Autodesk Inventor part; units mm, degrees
ref_plane "YZ Plane" through (0, 0, 0) normal (1, 0, 0) x (0, 1, 0)
ref_plane "XZ Plane" through (0, 0, 0) normal (0, 1, 0) x (-1, 0, 0)
ref_plane "XY Plane" through (0, 0, 0) normal (0, 0, 1) x (1, 0, 0)
sketch "スケッチ1" plane through (0, 0, 0) normal (0, 0, 1) x (1, 0, 0)
  line L0 (-100, -100) -> (100, -100)
  line L1 (100, -100) -> (100, 100)
  line L2 (100, 100) -> (-100, 100)
  line L3 (-100, 100) -> (-100, -100)
  line L4 (-100, -100) -> (100, 100) construction
  line L5 (100, -100) -> (-100, 100) construction
  point P0 (0, 0)
  dimension "d0" = 200
  dimension "d1" = 200
extrude "押し出し1" add sketch "スケッチ1" along normal blind 2
sketch "スケッチ2" plane through (0, 0, 2) normal (0, 0, 1) x (1, 0, 0)
  line L0 (100, 100) -> (-100, 100)
  line L1 (100, 100) -> (70, 100)
  line L2 (70, 100) -> (70, 70)
  line L3 (70, 70) -> (100, 70)
  line L4 (100, 70) -> (100, 100)
  line L5 (-100, -100) -> (100, -100)
  line L6 (-100, 100) -> (-100, -100)
  line L7 (-100, 100) -> (-70, 100)
  line L8 (-70, 100) -> (-70, 70)
  line L9 (-70, 70) -> (-100, 70)
  line L10 (-100, 70) -> (-100, 100)
  point P0 (0, 0)
  point P1 (-100, 70)
  dimension "d4" = 170
  dimension "d5" = 30
  dimension "d6" = 30
  dimension "d7" = 170
extrude "押し出し2" cut sketch "スケッチ2" against normal blind 2
sketch "スケッチ3" plane through (0, 0, 0) normal (0, 0, -1) x (-1, 0, 0)
  line L0 (-70, 100) -> (70, 100)
  point P0 (0, 0)
  point P1 (-35.7932, 78)
  point P2 (37.7411, 78)
  point P3 (-61, 89.1596)
  point P4 (61, 89.1596)
  point P5 (-50, 82.5)
  point P6 (-30, 82.5)
  point P7 (-10, 82.5)
  point P8 (0.0001, 82.5183)
  point P9 (10, 82.5545)
  point P10 (30, 82.5545)
  point P11 (50, 82.5545)
  point P12 (51.6496, 93.6869)
  dimension "d10" = 22
  dimension "d11" = 61
  dimension "d12" = 61
  dimension "d13" = 17.5
  dimension "d14" = 11
  dimension "d15" = 31
  dimension "d16" = 51
  dimension "d17" = 71
  dimension "d18" = 91
  dimension "d19" = 111
hole "穴1" at (50, 82.5, 0) at (30, 82.5, 0) at (10, 82.5, 0) at (-10, 82.5545, 0) at (-30, 82.5545, 0) at (-50, 82.5545, 0) at (-0.0001, 82.5183, 0) direction (0, 0, 1) diameter 3.4 end through all
sketch "スケッチ4" plane through (0, 0, 0) normal (0, 0, -1) x (-1, 0, 0)
  line L0 (-70, 70) -> (-100, 70)
  line L1 (-100, -100) -> (-100, 70)
  line L2 (100, 70) -> (100, -100)
  line L3 (100, 70) -> (70, 70)
  point P0 (0, 0)
  point P1 (-90, 55)
  point P2 (-66, 55)
  point P3 (-90, 25)
  point P4 (-66, 25)
  point P5 (90, 58)
  point P6 (66, 58)
  point P7 (90, 12.16)
  point P8 (66, 12.16)
  dimension "d27" = 15
  dimension "d28" = 15
  dimension "d29" = 10
  dimension "d30" = 24
  dimension "d31" = 10
  dimension "d32" = 30
  dimension "d33" = 30
  dimension "d34" = 24
  dimension "d35" = 10
  dimension "d36" = 12
  dimension "d37" = 24
  dimension "d38" = 10
  dimension "d39" = 24
hole "穴2" at (66, 25, 0) at (90, 25, 0) at (66, 55, 0) at (90, 55, 0) direction (0, 0, 1) diameter 3.4 end through all
sketch "スケッチ5" plane through (0, 0, 0) normal (0, 0, -1) x (-1, 0, 0)
  point P0 (0, 0)
sketch "スケッチ6" plane through (0, 0, 0) normal (0, 0, -1) x (-1, 0, 0)
  line L0 (100, 70) -> (70, 70)
  line L1 (100, 70) -> (100, -100)
  point P0 (0, 0)
  point P1 (90, 55)
  point P2 (66, 55)
  point P3 (90, 25)
  point P4 (66, 25)
  dimension "d47" = 15
  dimension "d48" = 15
  dimension "d49" = 10
  dimension "d50" = 24
  dimension "d51" = 10
  dimension "d52" = 24
  dimension "d53" = 30
  dimension "d54" = 30
hole "穴3" at (-90, 25, 0) at (-66, 25, 0) at (-66, 55, 0) at (-90, 55, 0) direction (0, 0, 1) diameter 3.4 end through all
sketch "スケッチ7" plane through (0, 0, 0) normal (0, 0, -1) x (-1, 0, 0)
  point P0 (0, 0)
sketch "スケッチ8" plane through (0, 0, 0) normal (0, 0, -1) x (-1, 0, 0)
  line L0 (-100, -100) -> (-100, 70)
  line L1 (-70, 70) -> (-100, 70)
  line L2 (100, 70) -> (70, 70)
  line L3 (100, 70) -> (100, -100)
  point P0 (0, 0)
  point P1 (-95, 65)
  point P2 (95, 65)
  dimension "d62" = 5
  dimension "d63" = 5
  dimension "d64" = 5
  dimension "d65" = 5
hole "穴4" at (95, 65, 0) at (-95, 65, 0) direction (0, 0, 1) diameter 3.4 end through all
sketch "スケッチ9" plane through (0, 0, 0) normal (0, 0, -1) x (-1, 0, 0)
  line L0 (-100, -100) -> (-100, 70)
  line L1 (100, -100) -> (-100, -100)
  line L2 (100, 70) -> (100, -100)
  point P0 (0, 0)
  point P1 (-95, -95)
  point P2 (95, -95)
  dimension "d73" = 5
  dimension "d74" = 5
  dimension "d75" = 5
  dimension "d76" = 5
hole "穴5" at (95, -95, 0) at (-95, -95, 0) direction (0, 0, 1) diameter 3.4 end through all
sketch "スケッチ10" plane through (0, 0, 0) normal (0, 0, -1) x (-1, 0, 0)
  circle A0 centre (-95, 65) radius 1.7
  line L0 (-100, -100) -> (-100, 70)
  line L1 (100, 70) -> (100, -100)
  point P0 (0, 0)
  point P1 (-95, -15)
  point P2 (95, -25)
  dimension "d84" = 80
  dimension "d85" = 5
  dimension "d86" = 5
hole "穴6" at (95, -15, 0) direction (0, 0, 1) diameter 3.4 end through all
sketch "スケッチ11" plane through (0, 0, 0) normal (0, 0, -1) x (-1, 0, 0)
  line L0 (-70, 100) -> (70, 100)
  point P0 (0, 0)
  point P1 (0, 0)
  point P2 (0, -10)
  dimension "d94" = 110
hole "穴7" at (0, -10, 0) direction (0, 0, 1) diameter 3.4 end through all
sketch "スケッチ12" plane through (0, 0, 0) normal (0, 0, -1) x (-1, 0, 0)
  line L0 (100, -100) -> (-100, -100)
  line L1 (100, 70) -> (100, -100)
  line L2 (-100, -100) -> (-100, 70)
  point P0 (0, 0)
  point P1 (-95, -80)
  point P2 (95, -80)
  dimension "d102" = 20
  dimension "d103" = 20
  dimension "d104" = 5
  dimension "d105" = 5
hole "穴8" at (95, -80, 0) at (-95, -80, 0) direction (0, 0, 1) diameter 3.4 end through all
sketch "スケッチ13" plane through (0, 0, 0) normal (0, 0, -1) x (-1, 0, 0)
  point P0 (0, 0)
sketch "スケッチ14" plane through (0, 0, 0) normal (0, 0, -1) x (-1, 0, 0)
  line L0 (100, 70) -> (100, -100)
  circle A0 centre (95, 65) radius 1.7
  point P0 (0, 0)
  point P1 (95, -15)
  dimension "d113" = 5
  dimension "d114" = 80
hole "穴9" at (-95, -15, 0) direction (0, 0, 1) diameter 3.4 end through all
sketch "スケッチ15" plane through (0, 0, 0) normal (0, 0, -1) x (-1, 0, 0)
  circle A0 centre (0, -10) radius 1.7
  point P0 (0, 0)
  point P1 (0, -3)
  dimension "d122" = 7
hole "穴10" at (0, -3, 0) direction (0, 0, 1) diameter 3.4 end through all
sketch "スケッチ16" plane through (0, 0, 2) normal (0, 0, 1) x (1, 0, 0)
  point P0 (0, 0)
  point P1 (-5, 24.9689)
  point P2 (5, 25)
  point P3 (5, 35)
  point P4 (-5, 34.9689)
  dimension "d130" = 5
  dimension "d131" = 5
  dimension "d132" = 10
  dimension "d133" = 10
  dimension "d134" = 5
  dimension "d135" = 5
hole "穴11" at (-5, 34.9689, 2) at (-5, 24.9689, 2) at (5, 25, 2) at (5, 35, 2) direction (0, 0, -1) diameter 2.459 depth 8.8 tip angle 118
sketch "スケッチ17" plane through (0, 0, 2) normal (0, 0, 1) x (1, 0, 0)
  point P0 (0, 0)
properties part number "20220522"
Part model, mm, in its own coordinate system. Give positions to 0.01 mm unless a question says otherwise; leave off trailing zeros. Loops run counter-clockwise (first coordinate to the right, second up) from the corner with the lowest first, then second, coordinate; pieces in that order, holes last. Notation, with made-up numbers: M -9.5,-38 L -5.5,-38 A33 cw -5.5,-6 Z; hole C 71.25,-19.5 d3. An arc over 180 degrees is marked long. Put each result on its own line as item: value. Start each with the question number.
1) Probe probe 1 along Y at (x, z) = (-95, 0.9); probe 2 along Y at (x, z) = (-66, 1.45); probe 3 along X at (y, z) = (-10, 0.4). List the from-to ranges inside material, lowest first.
2) Saw through at B-B (z = 1.25). State how many separate pieces and enclosed holes the cut face has, then the cut area to 3 significant figures.
3) Saw through at A-A (x = 81.5). List the corners of the cut face in (y, z), then the cut area to 3 significant figures.
4) Flat gauge pins, fed straight in: pin 1 (2.5 mm diameter, centred on x = 10, y = 82.5, fed in from -Z); pin 2 (1 mm diameter, centred on y = 91, z = 1.5, fed in from +X). Where does each tip first touch, or does it go through?
Numbers:
1. probe 1: -100 to -96.7, -93.3 to -81.7, -78.3 to -16.7, -13.3 to 63.3, 66.7 to 70
1. probe 2: -100 to 23.3, 26.7 to 53.3, 56.7 to 100
1. probe 3: -100 to -1.7, 1.7 to 100
2. separate pieces: 1
2. enclosed holes: 29
2. area: 38,000 mm^2
3. outline: M -100,0 L 70,0 L 70,2 L -100,2 Z
3. area: 340 mm^2
4. pin 1: through
4. pin 2: x = 70
